from build123d import *

# Parameters (mm, degrees)
EXTRUDE_1_DEPTH     = 44
SKETCH_2_R          = 1.5
CUT_EXTRUDE_1_DEPTH = 2
SKETCH_3_R          = 1.5
EXTRUDE_2_DEPTH     = 1
SKETCH_4_R          = 1.5
EXTRUDE_3_DEPTH     = 1


with BuildPart() as part:
    # 草圖1 → 填料-伸長1 (new body)
    with BuildSketch(Plane.XY):
        Polygon((5, -5), (13.5, -5), (13.5, 5), (-13.5, 5), (-13.5, -5), (-5, -5), (-5, 0), (5, 0), align=None)
    extrude(amount=EXTRUDE_1_DEPTH)

    # 草圖2 → 除料-伸長1 (cut)
    with BuildSketch(Plane(origin=(0, 5, 0), x_dir=(1, 0, 0), z_dir=(0, 1, 0))):
        with Locations(Location((-10, -32, 0), (0, 0, 270))):
            Circle(SKETCH_2_R)
        with Locations(Location((10, -32, 0), (0, 0, 90))):
            Circle(SKETCH_2_R)
        with Locations(Location((10, -12, 0), (0, 0, 270))):
            Circle(SKETCH_2_R)
        with Locations(Location((-10, -12, 0), (0, 0, 90))):
            Circle(SKETCH_2_R)
    extrude(amount=-CUT_EXTRUDE_1_DEPTH, mode=Mode.SUBTRACT)

    # 草圖3 → 填料-伸長2 (add)
    with BuildSketch(Plane.XY.offset(44)):
        with Locations((-8, -0.28409819)):
            Circle(SKETCH_3_R)
        with Locations(Location((8, -0.28409819, 0), (0, 0, 180))):
            Circle(SKETCH_3_R)
    extrude(amount=EXTRUDE_2_DEPTH)

    # 草圖4 → 填料-伸長3 (add)
    with BuildSketch(Plane(origin=(0, 0, 0), x_dir=(-1, 0, 0), z_dir=(0, 0, -1))):
        with Locations(Location((-8, 0, 0), (0, 0, 180))):
            Circle(SKETCH_4_R)
        with Locations(Location((8, 0, 0), (0, 0, 180))):
            Circle(SKETCH_4_R)
    extrude(amount=EXTRUDE_3_DEPTH)


solid = part.part
Can you work these out from the model? Positions are in its coordinate system, mm. A direction names the side the tool comes from. Coordinates: 2 decimals unless noted, no trailing zeros. Loops run counter-clockwise (first coordinate to the right, second up) from the corner with the lowest first, then second, coordinate; pieces in that order, holes last. Notation, with made-up numbers: M 68.25,-40 L 106.25,-40 A29 ccw 106.25,-17 Z; hole C 53.25,35 d9. An arc over 180 degrees is marked long. Answer as CSV lines item,"result". Start each with the question number.
1. If I drill on probe 1 along X at (y, z) = (4.2, 12); probe 2 along X at (y, z) = (-1.75, 36.5); probe 3 along X at (y, z) = (3.5, 12.5), over which ranges is the centre line in solid material (lowest first)? Write a range as [from, to].
2. For faces 4 (the face through (10, 3, 12)), 5 (the face through (6.5, -0.07, -0.49)), 6 (the face through (5, -2, 22)), which set-ups out of +Z, -Z, +X, -X, +Y, -Y let a thin tool reach every point of the face, with its end or its side?
3. Suppose I cut it at C-C, the plane x = -10. List the corners of the cut face in (y, z) for me, plus the area to 3 significant figures.
4. For pin 1 Ø2 at (x, y) = (-4.5, 4) entering from +Z; pin 2 Ø0.9 at (x, z) = (10.5, 11.5) entering from +Y; pin 3 Ø3 at (x, y) = (2.5, 2) entering from -Z, each with a flat end and sliding along its axis, tell me the tip position at first contact or that it passes through.
5. Thinking about a two-plate mould opening in Z: for faces 1 (the face through (-5, -3, 22)), 2 (the face through (10, 3, 32)), 3 (the face through (-8, 0, 45)), which applies, +Z half, -Z half, draft (parallel to the pull), parting line (faces both ways), or undercut?
6. Suppose I cut it at B-B, the plane z = 32. List the corners of the cut face in (x, y) for me.
7. Suppose I cut it at D-D, the plane x = 8. List the corners of the cut face in (y, z) for me, plus the area to 3 significant figures.
8. Suppose I cut it at A-A, the plane y = 4.25. List the corners of the cut face in (x, z) for me, plus the area to 3 significant figures.
Output:
1,probe 1,"x = [-13.5, -11.5], [-8.5, 8.5], [11.5, 13.5]"
1,probe 2,"x = [-13.5, -5], [5, 13.5]"
1,probe 3,"x = [-13.5, -11.41], [-8.59, 8.59], [11.41, 13.5]"
2,face 4,"+Y"
2,face 5,"-Z"
2,face 6,"+Z, -Z, -Y"
3,outline,"M -5,0 L 5,0 L 5,10.5 L 3,10.5 L 3,13.5 L 5,13.5 L 5,30.5 L 3,30.5 L 3,33.5 L 5,33.5 L 5,44 L -5,44 Z"
3,area,"428 mm^2"
4,pin 1,"stops at z = 44"
4,pin 2,"stops at y = 3"
4,pin 3,"stops at z = 0"
5,face 1,"draft"
5,face 2,"undercut"
5,face 3,"+Z half"
6,outline,"M -13.5,-5 L -5,-5 L -5,0 L 5,0 L 5,-5 L 13.5,-5 L 13.5,5 L 11.5,5 L 11.5,3 L 8.5,3 L 8.5,5 L -8.5,5 L -8.5,3 L -11.5,3 L -11.5,5 L -13.5,5 Z"
7,outline,"M -5,0 L -1.5,0 L -1.5,-1 L 1.5,-1 L 1.5,0 L 5,0 L 5,44 L 1.22,44 L 1.22,45 L -1.78,45 L -1.78,44 L -5,44 Z"
7,area,"446 mm^2"
8,outline,"M -13.5,0 L 13.5,0 L 13.5,44 L -13.5,44 Z; hole C -10,12 d3; hole C -10,32 d3; hole C 10,12 d3; hole C 10,32 d3"
8,area,"1,160 mm^2"
